Read the model definition and answer for the solid it produces. Units are mm, in the model's axes. A direction names the side the tool comes from. Coordinates: 2 decimals unless noted, no trailing zeros. Write each loop counter-clockwise with the first axis right and the second up, starting at its lowest first coordinate (ties: lowest second). Pieces come first, ordered by that corner, then holes. Notation, with made-up numbers: (-23.5, -21) -> (-3.5, -21) arc R24 cw to (-3.5, -8) -> close; hole circle Ø7 at (45, 35). An arc over 180 degrees is marked (long way). Answer in a Markdown table with one row per item. Add a question column.
Item 1: Given pin 1 Ø1.5 at (y, z) = (111, -5) entering from -X; pin 2 Ø1.5 at (y, z) = (8.5, -3) entering from -X; pin 3 Ø2.5 at (x, z) = (28, -3) entering from -Y, each flat-ended and moving along its own axis, determine where each tip first touches the part or whether it passes through.
Item 2: Section A-A on y = 51.5 is taken. Write down the section's boundary in (x, z).
Item 3: Straight lines are drawn through the part: line 1 (Z direction, x = 209, y = 188.5); line 2 (Y direction, x = 113.5, z = -11.75); line 3 (X direction, y = 79, z = -16). For each, find the intervals that lie inside material, in ascending order. Write a range as from..to.
Item 4: Section D-D on y = 168 is taken. Write down the section's boundary in (x, z).
Item 5: Which of the six approach directions +Z, -Z, +X, -X, +Y, -Y give full straight-line access (tool end or side, diameter ignored) to faces 1 (the face through (217, 68, -13)), 2 (the face through (116, 43, -13)), 3 (the face through (17, 68, -13))?
Item 6: Section B-B on x = 175 is taken. Write down the section's boundary in (y, z), then the cut area to 3 significant figures.
Item 7: Section C-C on z = -13.5 is taken. Write down the section's boundary in (x, y), then the cut area to 3 significant figures.
```python
from build123d import *

# Parameters (mm, degrees)
PAD002_DEPTH = 1.5
PAD003_DEPTH = 6.5
SKETCH005_W  = 200
SKETCH005_H  = 50
PAD005_DEPTH = 19


with BuildPart() as part:
    # Sketch002 → Pad002 (new body)
    with BuildSketch(Plane.XY):
        with BuildLine():
            Line((1, 0), (366.9, 0))
            ThreePointArc((366.9, 0), (367.607107, 0.292893), (367.9, 1))
            Line((367.9, 1), (367.9, 221.4))
            ThreePointArc((367.9, 221.4), (367.607107, 222.107107), (366.9, 222.4))
            Line((366.9, 222.4), (1, 222.4))
            ThreePointArc((1, 222.4), (0.292893, 222.107107), (0, 221.4))
            Line((0, 221.4), (0, 1))
            ThreePointArc((0, 1), (0.292893, 0.292893), (1, 0))
        make_face()
    extrude(amount=-PAD002_DEPTH)

    # Sketch003 → Pad003 (join)
    with BuildSketch(Plane.XY):
        Polygon((6.5, 12.5), (6.5, 218.4), (365.4, 218.4), (365.4, 12.5), (330.4, 12.5), (330.4, 1), (41.5, 1), (41.5, 12.5), align=None)
    extrude(amount=-PAD003_DEPTH)

    # Sketch005 → Pad005 (join)
    with BuildSketch(Plane.XY):
        with Locations((117, 68)):
            Rectangle(SKETCH005_W, SKETCH005_H)
    extrude(amount=-PAD005_DEPTH)


solid = part.part
```
Results below:
| question | item | result |
|---|---|---|
| 1 | pin 1 | stops at x = 6.5 |
| 1 | pin 2 | stops at x = 41.5 |
| 1 | pin 3 | stops at y = 12.5 |
| 2 | outline | (0, -1.5) -> (6.5, -1.5) -> (6.5, -6.5) -> (17, -6.5) -> (17, -19) -> (217, -19) -> (217, -6.5) -> (365.4, -6.5) -> (365.4, -1.5) -> (367.9, -1.5) -> (367.9, 0) -> (0, 0) -> close |
| 3 | line 1 | z = -6.5..0 |
| 3 | line 2 | y = 43..93 |
| 3 | line 3 | x = 17..217 |
| 4 | outline | (0, -1.5) -> (6.5, -1.5) -> (6.5, -6.5) -> (365.4, -6.5) -> (365.4, -1.5) -> (367.9, -1.5) -> (367.9, 0) -> (0, 0) -> close |
| 5 | face 1 | -Z, +X, +Y, -Y |
| 5 | face 2 | -Z, +X, -X, -Y |
| 5 | face 3 | -Z, -X, +Y, -Y |
| 6 | outline | (0, -1.5) -> (1, -1.5) -> (1, -6.5) -> (43, -6.5) -> (43, -19) -> (93, -19) -> (93, -6.5) -> (218.4, -6.5) -> (218.4, -1.5) -> (222.4, -1.5) -> (222.4, 0) -> (0, 0) -> close |
| 6 | area | 2,050 mm2 |
| 7 | outline | (17, 43) -> (217, 43) -> (217, 93) -> (17, 93) -> close |
| 7 | area | 10,000 mm2 |
